from build123d import *

# Parameters (mm, degrees)
BOSS_EXTRUDE1_DEPTH = 26
SKETCH3_R           = 20.325
SKETCH3_R_2         = 18.5
CUT_EXTRUDE1_DEPTH  = 10
FILLET1_R           = 10
FILLET5_R           = 1
CUT_EXTRUDE2_DEPTH  = 16
SKETCH10_R          = 11.52
CUT_EXTRUDE4_DEPTH  = 75


with BuildPart() as part:
    # Sketch2 → Boss-Extrude1 (new, symmetric)
    with BuildSketch(Plane.XY):
        with BuildLine():
            Line((-27.5, -27.5), (-27.5, 0))
            Line((-27.5, 0), (27.5, 0))
            Line((27.5, 0), (27.5, -27.5))
            ThreePointArc((27.5, -27.5), (0, -55), (-27.5, -27.5))
        make_face()
    extrude(amount=BOSS_EXTRUDE1_DEPTH, both=True)

    # Sketch3 → Cut-Extrude1 (cut)
    with BuildSketch(Plane(origin=(0, 0, 0), x_dir=(1, 0, 0), z_dir=(0, 1, 0))):
        with Locations(Location((0, 0, 0), (0, 0, 270))):
            Circle(SKETCH3_R)
        with Locations(Location((0, 0, 0), (0, 0, 270))):
            Circle(SKETCH3_R_2, mode=Mode.SUBTRACT)
    extrude(amount=-CUT_EXTRUDE1_DEPTH, mode=Mode.SUBTRACT)

    # Fillet1
    fillet1_edges = [part.edges().sort_by_distance(p)[0] for p in [
        (-27.5, -13.75, 26),
        (0, -55, 26),
        (-27.5, -13.75, -26),
        (27.5, -13.75, -26),
        (0, -55, -26),
        (27.5, -13.75, 26),
    ]]
    fillet(fillet1_edges, radius=FILLET1_R)

    # Fillet5
    fillet5_edges = [part.edges().sort_by_distance(p)[0] for p in [
        (27.5, 0, 0),
        (0, 0, -26),
        (-27.5, 0, 0),
        (0, 0, 26),
        (-24.571067812, 0, 23.071067812),
        (-24.571067812, 0, -23.071067812),
        (24.571067812, 0, 23.071067812),
        (24.571067812, 0, -23.071067812),
    ]]
    fillet(fillet5_edges, radius=FILLET5_R)

    # Sketch7 → Cut-Extrude2 (cut, symmetric)
    with BuildSketch(Plane.XY):
        with BuildLine():
            Line((-0.011296589, -11.876404256), (-25.011296589, -11.876404256))
            Line((-25.011296589, -11.876404256), (-25.011296589, -36.876404256))
            ThreePointArc((-25.011296589, -36.876404256), (-0.011296589, -61.876404256), (24.988703411, -36.876404256))
            Line((24.988703411, -36.876404256), (24.988703411, -11.876404256))
            Line((24.988703411, -11.876404256), (-0.011296589, -11.876404256))
        make_face()
    extrude(amount=CUT_EXTRUDE2_DEPTH, both=True, mode=Mode.SUBTRACT)

    # Sketch10 → Cut-Extrude4 (cut)
    with BuildSketch(Plane.XY.offset(26)):
        with Locations((0, -28.319318025)):
            Circle(SKETCH10_R)
    extrude(amount=-CUT_EXTRUDE4_DEPTH, mode=Mode.SUBTRACT)


solid = part.part
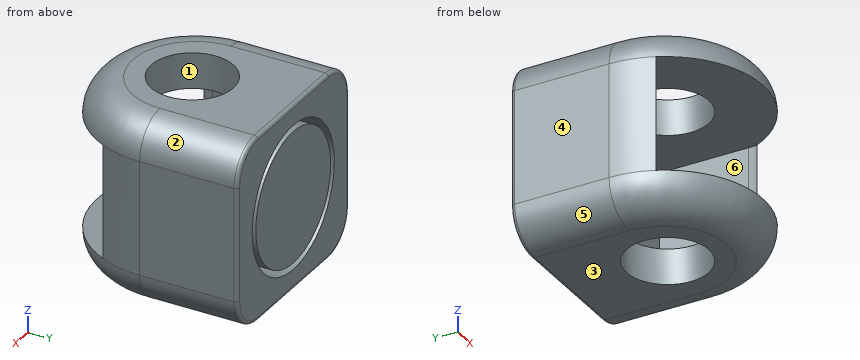
Geometry: final body of the model. Coordinates: model frame, mm. Face numbers are marked on the shaded views. A direction names the side the tool comes from. Give positions to 0.01 mm unless a question says otherwise; leave off trailing zeros. Write each loop counter-clockwise with the first axis right and the second up, starting at its lowest first coordinate (ties: lowest second). Pieces come first, ordered by that corner, then holes. Notation, with made-up numbers: (46.5, 15.25) -> (60.5, 15.25) arc R20 ccw to (60.5, 26.25) -> close; hole circle Ø3 at (70.25, 32). An arc over 180 degrees is marked (long way). Answer as a JSON object with one key per item and string values.
1. Cut plane B-B on x = 0. Output: boundary loops of the cut face in (y, z) (3 decimals), and give its area (3 significant figures).
Ans:
{"outline": "(-55, -16) arc R10 ccw to (-45, -26) -> (-39.839, -26) -> (-39.839, -16) -> close; (-55, 16) -> (-39.839, 16) -> (-39.839, 26) -> (-45, 26) arc R10 ccw to start; (-16.799, -26) -> (-1, -26) arc R1 ccw to (0, -25) -> (0, -20.325) -> (-10, -20.325) -> (-10, -18.5) -> (0, -18.5) -> (0, 18.5) -> (-10, 18.5) -> (-10, 20.325) -> (0, 20.325) -> (0, 25) arc R1 ccw to (-1, 26) -> (-16.799, 26) -> (-16.799, 16) -> (-11.876, 16) -> (-11.876, -16) -> (-16.799, -16) -> close", "area": "939 mm^2"}
2. Mould query, pull axis X, two halves, no side actions, for the marked faces 1, 2, 3 and 4. Classes: pulls with the +X half, pulls with the -X half, needs draft (parallel to the pull), parting line crosses it, or undercut.
Ans:
{"face 1": "undercut", "face 2": "pulls with the +X half", "face 3": "needs draft", "face 4": "pulls with the -X half"}
3. Cut plane C-C on z = 0. Output: boundary loops of the cut face in (x, y) (3 decimals), and give its area (3 significant figures).
Ans:
{"outline": "(-27.5, -27.5) arc R27.5 ccw to (-24.907, -39.157) arc R25 cw to (-25.011, -36.876) -> (-25.011, -11.876) -> (24.989, -11.876) -> (24.989, -36.876) arc R25 cw to (24.879, -39.217) arc R27.5 ccw to (27.5, -27.5) -> (27.5, -1) arc R1 ccw to (26.5, 0) -> (20.325, 0) -> (20.325, -10) -> (18.5, -10) -> (18.5, 0) -> (-18.5, 0) -> (-18.5, -10) -> (-20.325, -10) -> (-20.325, 0) -> (-26.5, 0) arc R1 ccw to (-27.5, -1) -> close", "area": "733 mm^2"}
4. Ray query, probe 1 along X at (y, z) = (-5.5, 0) (3 decimals); probe 2 along X at (y, z) = (-27, -11); probe 3 along Z at (x, y) = (16.5, -14.5). Return the intervals inside material, ascending. Write a range as from..to.
Ans:
{"probe 1": "x = -27.5..-20.325, -18.5..18.5, 20.325..27.5", "probe 2": "x = -27.5..-25.01, 24.99..27.5", "probe 3": "z = -26..-16, 16..26"}
5. Access query for the marked faces 5 and 6. Directions: +Z, -Z, +X, -X, +Y, -Y. A direction counts if a zero-diameter tool reaches every point of the face in a straight line with its end or side. Return the directions, or none.
Ans:
{"face 5": "-Z, -X, +Y, -Y", "face 6": "none"}
6. Contact query for flat-ended pins moving along their axis: pin 1 (1 mm diameter, centred on x = 17, z = 11, fed in from -Y); pin 2 (20.5 mm diameter, centred on x = 0, y = -28.32, fed in from +Z); pin 3 (6 mm diameter, centred on x = 22, y = -32.5, fed in from -Z); pin 4 (1 mm diameter, centred on x = 22, y = -41.5, fed in from +Z). Output: stop coordinate, or through.
Ans:
{"pin 1": "stops at y = -11.88", "pin 2": "passes through", "pin 3": "stops at z = -25.79", "pin 4": "stops at z = 21.9"}
7. Cut plane A-A on y = -5. Output: boundary loops of the cut face in (x, z) (3 decimals), and give its area (3 significant figures).
Ans:
{"outline": "(-27.5, -16) arc R10 ccw to (-17.5, -26) -> (17.5, -26) arc R10 ccw to (27.5, -16) -> (27.5, 16) arc R10 ccw to (17.5, 26) -> (-17.5, 26) arc R10 ccw to (-27.5, 16) -> close; circle Ø37 at (0, 0); hole circle Ø40.65 at (0, 0)", "area": "2,550 mm^2"}
8. Cut plane D-D on z = 13. Output: boundary loops of the cut face in (x, y), and give its area (3 significant figures).
Ans:
{"outline": "(-27.5, -27.5) arc R27.5 ccw to (-24.91, -39.16) arc R25 cw to (-25.01, -36.88) -> (-25.01, -11.88) -> (24.99, -11.88) -> (24.99, -36.88) arc R25 cw to (24.88, -39.22) arc R27.5 ccw to (27.5, -27.5) -> (27.5, -1) arc R1 ccw to (26.5, 0) -> (15.62, 0) -> (15.62, -10) -> (13.16, -10) -> (13.16, 0) -> (-13.16, 0) -> (-13.16, -10) -> (-15.62, -10) -> (-15.62, 0) -> (-26.5, 0) arc R1 ccw to (-27.5, -1) -> close", "area": "720 mm^2"}
